```python
from build123d import *

# Parameters (mm, degrees)
SKETCH2_W = 1.905
SKETCH2_H = 10.16


with BuildPart() as part:
    # Sweep1: sweep along a path in Sketch1
    with BuildLine(Plane(origin=(0, 0, 0), x_dir=(1, 0, 0), z_dir=(0, 1, 0))) as sweep1_path:
        Line((0, 15.24), (325.005160504, 15.24))
        ThreePointArc((325.005160504, 15.24), (340.245160504, 0), (325.005160504, -15.24))
        Line((325.005160504, -15.24), (0, -15.24))
        ThreePointArc((0, -15.24), (-15.24, 0), (0, 15.24))
    # Sketch2 → Sweep1 (sweep)
    with BuildSketch(Plane(origin=(0, 0, 0), x_dir=(0, 0, -1), z_dir=(1, 0, 0))):
        with Locations((-15.24, 0)):
            Rectangle(SKETCH2_W, SKETCH2_H)
    sweep(path=sweep1_path.line)


solid = part.part
```
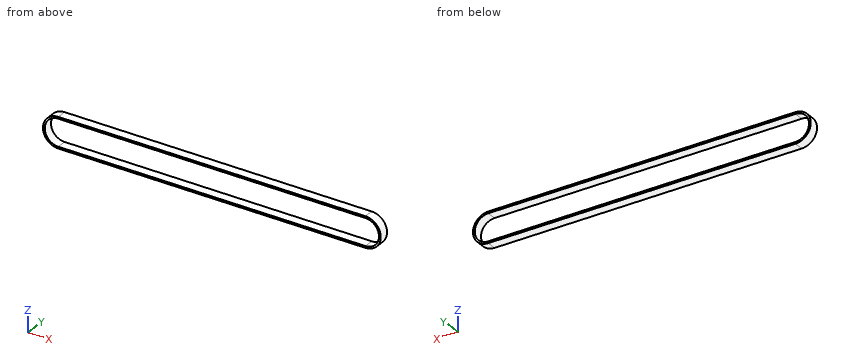
Geometry check sheet. Reference: the model listing, model coordinates, mm. Coordinates: 2 decimals unless noted, no trailing zeros. Order: outer loops, then holes, each group sorted by start corner. A loop starts at its lowest first (then second) coordinate and runs counter-clockwise, first axis right, second up. Notation, with made-up numbers: (9, 30) - (62, 30) arc R17 ccw to (62, 43) - close; hole circle Ø2 at (81, 37.25). An arc over 180 degrees is marked (long way). Use one line per item in the form item = value.
1. Section check C-C (y = 2). Record the boundary of the cut face in (x, z) (1 decimal), then the cut area to 3 significant figures.
Here are the results:
outline = (0, -16.2) - (325, -16.2) arc R16.2 ccw to (325, 16.2) - (0, 16.2) arc R16.2 ccw to start; hole (0, -14.3) - (325, -14.3) arc R14.3 ccw to (325, 14.3) - (0, 14.3) arc R14.3 ccw to start
area = 1,420 mm²
2. Section check B-B (z = -5.5). Record the boundary of the cut face in (x, y), then the cut area to 3 significant figures.
Here are the results:
outline = (-15.23, -5.08) - (-13.19, -5.08) - (-13.19, 5.08) - (-15.23, 5.08) - close; (338.19, -5.08) - (340.23, -5.08) - (340.23, 5.08) - (338.19, 5.08) - close
area = 41.5 mm²
3. Section check A-A (x = 102). Record the boundary of the cut face in (y, z), then the cut area to 3 significant figures.
Here are the results:
outline = (-5.08, -16.19) - (5.08, -16.19) - (5.08, -14.29) - (-5.08, -14.29) - close; (-5.08, 14.29) - (5.08, 14.29) - (5.08, 16.19) - (-5.08, 16.19) - close
area = 38.7 mm²
4. Scan lines: line 1 (Z direction, x = 84, y = -3.5); line 2 (X direction, y = 2, z = 1); line 3 (X direction, y = -4, z = 3.5). Record each from-to range of solid material in increasing order.
Here are the results:
line_1 = -16.19 to -14.29, 14.29 to 16.19
line_2 = -16.16 to -14.25, 339.26 to 341.17
line_3 = -15.81 to -13.85, 338.86 to 340.81
5. Gauge pin test, flat ends, axial feed: pin 1 (12 mm diameter, centred on x = 34, z = 8, fed in from -Y); pin 2 (1 mm diameter, centred on y = 0, z = -7.5, fed in from +X); pin 3 (1.5 mm diameter, centred on y = -2, z = -7, fed in from +X). Record the tip position at first contact, or that the pin passes through.
Here are the results:
pin_1 = through
pin_2 = 339.61
pin_3 = 339.94
